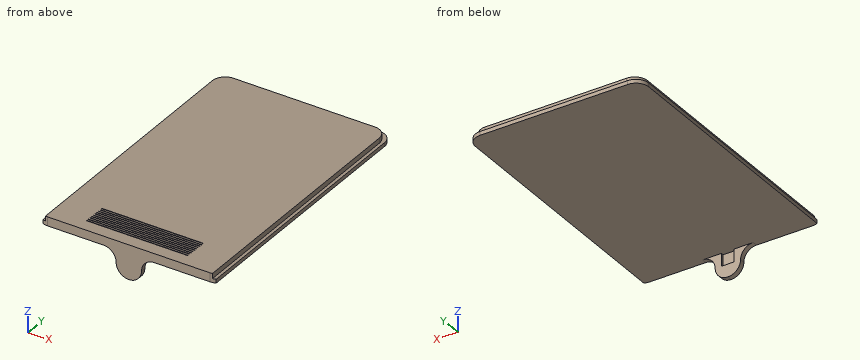
```python
from build123d import *

# Parameters (mm, degrees)
F1_DEPTH  = 106
F2_W      = 68.25
F2_H      = 1.5
F3_DEPTH  = 1.25
F4_R      = 5
F6_DEPTH  = 25
F7_W      = 10
F7_H      = 10
F8_DEPTH  = 2
F9_R      = 4.99999
F10_W     = 5
F10_H     = 5
F11_DEPTH = 1
F12_W     = 40
F12_H     = 0.25
F13_DEPTH = 1


# Not quite as in the source:
# - a fillet or chamfer is up to 0.001 mm smaller than in the source, because OpenCascade refuses the exact size


with BuildPart() as f1:
    # F0 (on Front) → F1 (new body)
    with BuildSketch(Plane.XZ):
        Polygon((32.875, 1.5), (32.875, 3.5), (-32.875, 3.5), (-32.875, 1.5), (-34.125, 1.5), (-34.125, 0), (34.125, 0), (34.125, 1.5), align=None)
    extrude(amount=-F1_DEPTH)

    # F2 (on face) → F3 (join)
    with BuildSketch(Plane(origin=(0, 106, 0), x_dir=(-1, 0, 0), z_dir=(0, 1, 0))):
        with Locations((0, 0.75)):
            Rectangle(F2_W, F2_H)
    extrude(amount=F3_DEPTH)

    # F4
    f4_edges = [f1.edges().sort_by_distance(p)[0] for p in [
        (34.125, 107.25, 0.75),
        (-34.125, 107.25, 0.75),
        (-32.875, 106, 2.5),
        (32.875, 106, 2.5),
    ]]
    fillet(f4_edges, radius=F4_R)

    # F5 (on Top) → F6 (cut)
    with BuildSketch(Plane.XY):
        with BuildLine():
            ThreePointArc((-32, 0), (-35.5355339059, 1.4644660941), (-37, 5))
            Line((-37, 5), (-47.4459486902, 5.1317643374))
            Line((-47.4459486902, 5.1317643374), (-32.4784885049, -8.2395952195))
            Line((-32.4784885049, -8.2395952195), (-32, 0))
        make_face()
        with BuildLine():
            Line((47.8749121428, 4.8458835855), (37, 4.9999998882))
            ThreePointArc((37, 4.9999998882), (35.5355339059, 1.4644659823), (32, -1.118e-07))
            Line((32, -1.118e-07), (31.699370116, -9.054190591))
            Line((31.699370116, -9.054190591), (47.8749121428, 4.8458835855))
        make_face()
    extrude(amount=F6_DEPTH, mode=Mode.SUBTRACT)

    # F7 (on face) → F8 (join)
    with BuildSketch(Plane.XZ):
        with Locations((0, -5)):
            Rectangle(F7_W, F7_H)
    extrude(amount=-F8_DEPTH)

    # F9 (radius 5 in the source; OpenCascade refuses exactly that, so slightly less here)
    f9_edges = [f1.edges().sort_by_distance(p)[0] for p in [
        (5, 1, 0),
        (-5, 1, 0),
        (-5, 1, -10),
        (5, 1, -10),
    ]]
    fillet(f9_edges, radius=F9_R)

    # F10 (on face) → F11 (cut)
    with BuildSketch(Plane(origin=(0, 2, 0), x_dir=(-1, 0, 0), z_dir=(0, 1, 0))):
        with Locations((0, -2.5)):
            Rectangle(F10_W, F10_H)
    extrude(amount=-F11_DEPTH, mode=Mode.SUBTRACT)

    # F12 (on face) → F13 (cut)
    with BuildSketch(Plane.XY.offset(3.5)):
        with Locations((0, 5.125)):
            Rectangle(F12_W, F12_H)
        with Locations((0.0169467185, 6.1248563941)):
            Rectangle(F12_W, F12_H)
        with Locations((0.0338934371, 7.1247127881)):
            Rectangle(F12_W, F12_H)
        with Locations((0.0508401556, 8.1245691822)):
            Rectangle(F12_W, F12_H)
        with Locations((0.0677868742, 9.1244255762)):
            Rectangle(F12_W, F12_H)
        with Locations((0.0847335927, 10.1242819703)):
            Rectangle(F12_W, F12_H)
        with Locations((0.1016803113, 11.1241383643)):
            Rectangle(F12_W, F12_H)
        with Locations((0.1186270298, 12.1239947584)):
            Rectangle(F12_W, F12_H)
        with Locations((0.1355737483, 13.1238511524)):
            Rectangle(F12_W, F12_H)
        with Locations((0.1525204669, 14.1237075465)):
            Rectangle(F12_W, F12_H)
    extrude(amount=-F13_DEPTH, mode=Mode.SUBTRACT)


solid = f1.part
```
Input: part model. Units: mm. Frame: model coordinates. Give positions to 0.01 mm unless a question says otherwise; leave off trailing zeros. Order: outer loops, then holes, each group sorted by start corner. A loop starts at its lowest first (then second) coordinate and runs counter-clockwise, first axis right, second up. Notation, with made-up numbers: (-26, -36) - (24, -36) arc R16 ccw to (24, -6) - close; hole circle Ø11 at (-4.75, 55). An arc over 180 degrees is marked (long way). One line per item, written item: value.
1. Line query: probe 1 along Z at (x, y) = (-17, 80); probe 2 along Y at (x, z) = (-27.5, 3); probe 3 along Y at (x, z) = (1, -7.5). Output: solid intervals per line, ascending.
Determined:
probe 1: 0 to 3.5
probe 2: 0 to 106
probe 3: 0 to 2
2. Pin query (flat end, axial travel): pin 1 Ø0.8 at (y, z) = (1.5, -3.5) entering from -X; pin 2 Ø2 at (x, y) = (-14, 86) entering from -Z; pin 3 Ø0.5 at (x, z) = (6, 3) entering from +Y. Return the tip coordinate at first contact, or that it passes through.
Determined:
pin 1: x = -5.38
pin 2: z = 0
pin 3: y = 106
3. Cut plane A-A, the plane y = 91. Output: boundary loops of the cut face in (x, z) (3 decimals), and give its area (3 significant figures).
Determined:
outline: (-34.125, 0) - (34.125, 0) - (34.125, 1.5) - (32.875, 1.5) - (32.875, 3.5) - (-32.875, 3.5) - (-32.875, 1.5) - (-34.125, 1.5) - close
area: 234 mm2
4. Cut plane B-B, the plane x = 22. Output: boundary loops of the cut face in (y, z).
Determined:
outline: (0, 0) - (107.25, 0) - (107.25, 1.5) - (106, 1.5) - (106, 3.5) - (0, 3.5) - close
5. Cut plane C-C, the plane z = -7.5. Output: boundary loops of the cut face in (x, y), and give its area (3 significant figures).
Determined:
outline: (-4.33, 0) - (4.33, 0) - (4.33, 2) - (-4.33, 2) - close
area: 17.3 mm2
